Geometry: final body of the model. Coordinates: model frame, mm. A direction names the side the tool comes from. Round coordinates to 2 decimals unless told otherwise and drop trailing zeros. Loops run counter-clockwise (first coordinate to the right, second up) from the corner with the lowest first, then second, coordinate; pieces in that order, holes last. Notation, with made-up numbers: (86.25, 41.5) - (103.25, 41.5) arc R15 ccw to (103.25, 55.5) - close; hole circle Ø1 at (-6.5, 71.25). An arc over 180 degrees is marked (long way). Answer as a JSON object with one key per item and string values. Group by question number.
Item 1: Draft query along X for faces 1 (the face through (60.785, 2.576, -31.948)), 2 (the face through (35.54, 2.5, -50.01)), 3 (the face through (85.61, 2.5, -22.94)). Return one class per face: released by +X, released by -X, zero draft, split by the parting line, or undercut.
Item 2: Section D-D (z = -84.5). Return the cut outline in (x, y).
Item 3: Section C-C (x = 59). Return the cut outline in (y, z), plus the area to 3 significant figures.
Item 4: Section A-A (z = -48). Return the cut outline in (x, y).
Item 5: First-contact query: pin 1 (2 mm diameter, centred on x = 53.5, y = 1.5, fed in from -Z); pin 2 (2 mm diameter, centred on y = 2, z = -71.5, fed in from -X); pin 3 (2 mm diameter, centred on y = 4, z = -39, fed in from +X). Flat tips, straight axial feed; report the tip coordinate or a pass-through.
Item 6: Line query: line 1 (X direction, y = 4.8, z = -49); line 2 (X direction, y = 1.3, z = -67.5); line 3 (Z direction, x = 35, y = 2.15). Output: solid intervals per line, ascending.
Item 7: Reachability of faces 4 (the face through (41.003, 2.576, -48.188)), 5 (the face through (48.137, 2.576, -40.953)), 6 (the face through (32.05, 2.58, -60.68)), 7 (the face through (49.91, 2.5, -35.64)) from +Z, -Z, +X, -X, +Y, -Y: full face, straight path, thin tool, end or side. Return the list, or none.
Item 8: Section B-B (y = 2.5). Return the cut outline in (x, z), plus the area to 4 significant figures.
```python
from build123d import *

# Parameters (mm, degrees)
BOSS_EXTRUDE1_DEPTH      = 5.08
M3_CLEARANCE_HOLE1_D     = 3.4
M3_CLEARANCE_HOLE1_DEPTH = 11.938
M3_CLEARANCE_HOLE1_TIP   = 1.021463052
CUT_EXTRUDE1_REACH       = 7.08


with BuildPart() as part:
    # Sketch1 → Boss-Extrude1 (new body)
    with BuildSketch(Plane(origin=(0, 0, 0), x_dir=(1, 0, 0), z_dir=(0, 1, 0))):
        with BuildLine():
            Line((27.939515919, 104.271692948), (18.0785103, 67.469918966))
            Line((18.0785103, 67.469918966), (67.469918966, 18.0785103))
            Line((67.469918966, 18.0785103), (104.271692948, 27.939515919))
            ThreePointArc((104.271692948, 27.939515919), (76.332177029, 76.332177029), (27.939515919, 104.271692948))
        make_face()
    extrude(amount=BOSS_EXTRUDE1_DEPTH)

    # M3 Clearance Hole1
    with Locations(Plane(origin=(0, 5.08, 0), x_dir=(1, 0, 0), z_dir=(0, 1, 0))):
        with Locations((70.944023356, 70.944023356)):
            Hole(M3_CLEARANCE_HOLE1_D / 2, depth=M3_CLEARANCE_HOLE1_DEPTH)
            with Locations((0, 0, -(M3_CLEARANCE_HOLE1_DEPTH + M3_CLEARANCE_HOLE1_TIP / 2))):  # 118° drill point
                Cone(0, M3_CLEARANCE_HOLE1_D / 2, M3_CLEARANCE_HOLE1_TIP, mode=Mode.SUBTRACT)

    # Sketch5 → Cut-Extrude1 (cut, up to next)
    with BuildSketch(Plane(origin=(0, 5.08, 0), x_dir=(1, 0, 0), z_dir=(0, 1, 0)), mode=Mode.PRIVATE) as cut_extrude1_sk1:
        Polygon((64.326829324, 28.40580484), (57.142624427, 35.590009736), (53.550521979, 31.997907288), (60.734726875, 24.813702391), align=None)
    cut_extrude1_tool1 = extrude(cut_extrude1_sk1.sketch, amount=-CUT_EXTRUDE1_REACH, mode=Mode.PRIVATE) & part.part
    add(cut_extrude1_tool1.solids().sort_by_distance((58.938676, 5.08, -30.201856))[0], mode=Mode.SUBTRACT)
    # Sketch5 → Cut-Extrude1 (cut, up to next)
    with BuildSketch(Plane(origin=(0, 5.08, 0), x_dir=(1, 0, 0), z_dir=(0, 1, 0)), mode=Mode.PRIVATE) as cut_extrude1_sk2:
        Polygon((49.95841953, 42.774214633), (42.774214633, 49.95841953), (39.182112185, 46.366317082), (46.366317082, 39.182112185), align=None)
    cut_extrude1_tool2 = extrude(cut_extrude1_sk2.sketch, amount=-CUT_EXTRUDE1_REACH, mode=Mode.PRIVATE) & part.part
    add(cut_extrude1_tool2.solids().sort_by_distance((44.570266, 5.08, -44.570266))[0], mode=Mode.SUBTRACT)
    # Sketch5 → Cut-Extrude1 (cut, up to next)
    with BuildSketch(Plane(origin=(0, 5.08, 0), x_dir=(1, 0, 0), z_dir=(0, 1, 0)), mode=Mode.PRIVATE) as cut_extrude1_sk3:
        Polygon((24.813702391, 60.734726875), (31.997907288, 53.550521979), (35.590009736, 57.142624427), (28.40580484, 64.326829324), align=None)
    cut_extrude1_tool3 = extrude(cut_extrude1_sk3.sketch, amount=-CUT_EXTRUDE1_REACH, mode=Mode.PRIVATE) & part.part
    add(cut_extrude1_tool3.solids().sort_by_distance((30.201856, 5.08, -58.938676))[0], mode=Mode.SUBTRACT)


solid = part.part
```
Values:
{
 "1": {"face 1": "undercut", "face 2": "released by -X", "face 3": "released by +X"},
 "2": {"outline": "(22.64, 0) - (67.18, 0) - (67.18, 5.08) - (22.64, 5.08) - close"},
 "3": {"outline": "(0, -90.4) - (5.08, -90.4) - (5.08, -33.73) - (0, -33.73) - close", "area": "288 mm^2"},
 "4": {"outline": "(37.55, 0) - (40.82, 0) - (40.82, 5.08) - (37.55, 5.08) - close; (44.73, 0) - (96.69, 0) - (96.69, 5.08) - (44.73, 5.08) - close"},
 "5": {"pin 1": "stops at z = -94.32", "pin 2": "stops at x = 18.89", "pin 3": "stops at x = 101.04"},
 "6": {"line 1": "x = 36.55 to 41.82, 43.73 to 96.19", "line 2": "x = 18.09 to 84.24", "line 3": "z = -102.12 to -57.73, -56.55 to -50.55"},
 "7": {"face 4": "+Z, +Y, -Y", "face 5": "-X, +Y, -Y", "face 6": "+Y, -Y", "face 7": "+Z, -X, +Y, -Y"},
 "8": {"outline": "(18.08, -67.47) - (27.94, -104.27) arc R107.95 ccw to (104.27, -27.94) - (67.47, -18.08) - (60.73, -24.81) - (64.33, -28.41) - (57.14, -35.59) - (53.55, -32) - (46.37, -39.18) - (49.96, -42.77) - (42.77, -49.96) - (39.18, -46.37) - (32, -53.55) - (35.59, -57.14) - (28.41, -64.33) - (24.81, -60.73) - close; hole circle Ø3.4 at (70.94, -70.94)", "area": "3,825 mm^2"}
}
